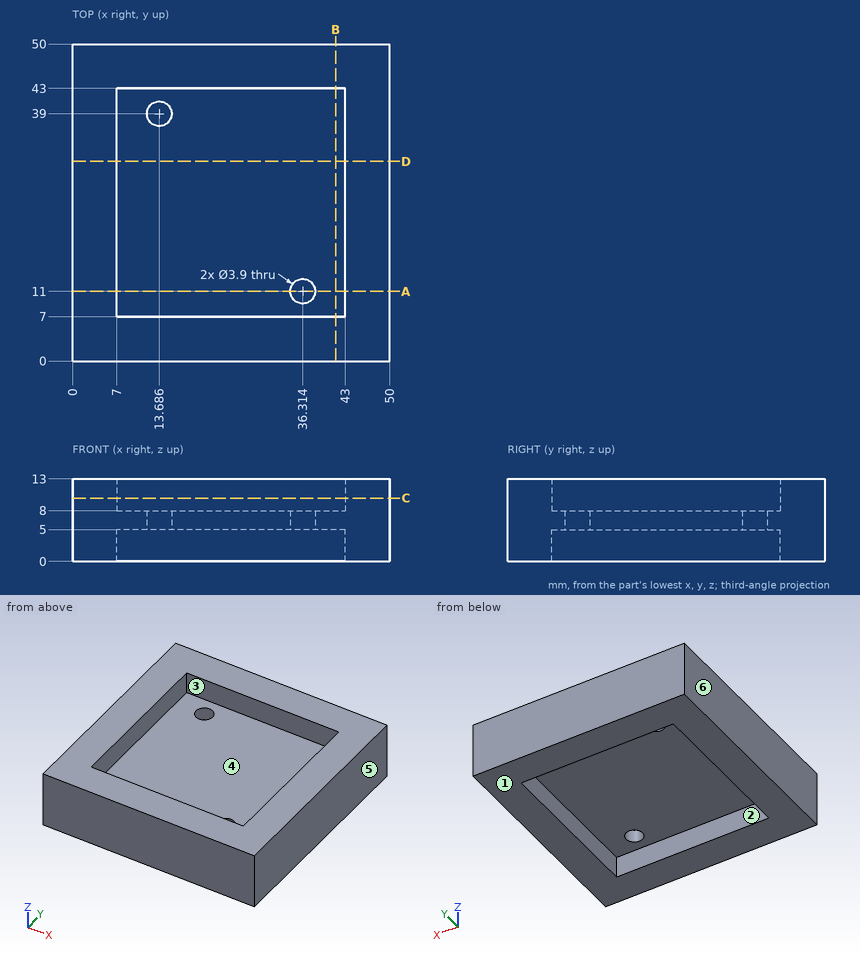
Answer from the drawing. Dimensions are ordinates in mm from the lowest x, y and z of the part. A direction names the side the tool comes from. Give positions to 0.01 mm unless a question says otherwise; leave off trailing zeros. Loops run counter-clockwise (first coordinate to the right, second up) from the corner with the lowest first, then second, coordinate; pieces in that order, holes last.
Item 1: A cutting plane is placed at B-B (x = 41.5). Give the vertices of the cut face in (y, z), then the cut area to 3 significant figures.
Derived:
outline: (0, 0) - (7, 0) - (7, 5) - (43, 5) - (43, 0) - (50, 0) - (50, 13) - (43, 13) - (43, 8) - (7, 8) - (7, 13) - (0, 13) - close
area: 290 mm2
Item 2: A cutting plane is placed at C-C (z = 10). Give the vertices of the cut face in (x, y).
Derived:
outline: (0, 0) - (50, 0) - (50, 50) - (0, 50) - close; hole (7, 7) - (43, 7) - (43, 43) - (7, 43) - close
Item 3: Each of these flat-tipped pins is pushed along its axis until it touches: pin 1 Ø1.5 at (x, y) = (14.5, 35) entering from +Z; pin 2 Ø4.5 at (x, y) = (13.69, 39) entering from -Z. Where does it stop, or does it pass through?
Derived:
pin 1: stops at z = 8
pin 2: stops at z = 5
Item 4: A cutting plane is placed at A-A (y = 11). Give the vertices of the cut face in (x, z).
Derived:
outline: (0, 0) - (7, 0) - (7, 5) - (34.36, 5) - (34.36, 8) - (7, 8) - (7, 13) - (0, 13) - close; (38.26, 5) - (43, 5) - (43, 0) - (50, 0) - (50, 13) - (43, 13) - (43, 8) - (38.26, 8) - close
Item 5: A tool of negligible diameter and unlimited length cuts with its end or side. For the marked faces 1 and 2, from which of +Z, -Z, +X, -X, +Y, -Y can it reach the whole face along a straight path? Write none if from no direction.
Derived:
face 1: -Z, +X, -X, +Y, -Y
face 2: -Z
Item 6: Determine the mould class of the marked faces 3, 4, 5 and 6 for opening direction X: +X half, -X half, draft (parallel to the pull), parting line (faces both ways), or undercut.
Derived:
face 3: undercut
face 4: undercut
face 5: +X half
face 6: -X half
Item 7: Find the intervals of material crossed by line 1 along Y through (x, z) = (30, 0.5); line 2 along Z through (x, y) = (32, 36), in increasing order.
Derived:
line 1: y = 0 to 7, 43 to 50
line 2: z = 5 to 8
